Geometry: final body of the model. Coordinates: model frame, mm. A direction names the side the tool comes from. Round coordinates to 2 decimals unless told otherwise and drop trailing zeros. Write each loop counter-clockwise with the first axis right and the second up, starting at its lowest first coordinate (ties: lowest second). Pieces come first, ordered by that corner, then holes. Notation, with made-up numbers: M 61,20 L 106,20 A27 cw 106,38 Z; hole C 75.5,-35 d6. An arc over 180 degrees is marked long. Use one line per item in the form item = value. Start each with the question number.
Item 1: Pull-direction query (Z, two-part tool) for faces 1 (the flat face through (-27, 49, -12.5)), 2 (the flat face through (-1, 60, 10)), 3 (the flat face through (-1, 59.1, 0)), 4 (the flat face through (-27, 49, 12.5)); classes: pulls with the +Z half, pulls with the -Z half, needs draft (parallel to the pull), parting line crosses it, or undercut.
Item 2: Reachability of faces 5 (the flat face through (-60, -1, 0)), 6 (the cylindrical face through (58.797, 58.859, 9.712)), 7 (the flat face through (-56, 57, 0)), 8 (the flat face through (-0.3, 59.4, -7)), 9 (the flat face through (58, 55.1, 0)) from +Z, -Z, +X, -X, +Y, -Y: full face, straight path, thin tool, end or side. Return the list, or none.
Item 3: Ray query, probe 1 along Y at (x, z) = (15, -5.75); probe 2 along X at (y, z) = (50, -4.75); probe 3 along Y at (x, z) = (5, 11). Return the intervals inside material, ascending.
Item 4: Section query B-B (x = 0). Return loops of the section in (y, z), and give its area (3 significant figures).
Item 5: Pin query (flat end, axial travel): pin 1 Ø2 at (y, z) = (56.5, 2) entering from -X; pin 2 Ø4 at (x, y) = (-52.5, 52.5) entering from -Z; pin 3 Ø2 at (x, z) = (58.5, 0.5) entering from +Y; pin 4 Ø4 at (x, z) = (2.5, -4.5) entering from +Y. Return the tip coordinate at first contact, or that it passes through.
Item 6: Section query C-C (z = 5). Return loops of the section in (x, y), and give its area (3 significant figures).
Item 7: Section query D-D (x = 52.5). Return loops of the section in (y, z), and give its area (3 significant figures).
Item 8: Section query A-A (y = 0). Return loops of the section in (x, z), and give its area (3 significant figures).
Autodesk Inventor part; units mm, degrees
ref_plane "YZ Plane" through (0, 0, 0) normal (1, 0, 0) x (0, 1, 0)
ref_plane "XZ Plane" through (0, 0, 0) normal (0, 1, 0) x (-1, 0, 0)
ref_plane "XY Plane" through (0, 0, 0) normal (0, 0, 1) x (1, 0, 0)
sketch "Sketch1" plane through (0, 0, 0) normal (0, 0, 1) x (1, 0, 0)
  line L0 (-56, 60) -> (56, 60)
  line L1 (60, 56) -> (60, -56)
  line L2 (56, -60) -> (-56, -60)
  line L3 (-60, -56) -> (-60, 56)
  line L4 (-60, 60) -> (60, -60) construction
  line L5 (60, 60) -> (-60, -60) construction
  circle A0 centre (0, 0) radius 55
  line L6 (-52.5, 52.5) -> (52.5, 52.5) construction
  line L7 (52.5, 52.5) -> (52.5, -52.5) construction
  line L8 (52.5, -52.5) -> (-52.5, -52.5) construction
  line L9 (-52.5, -52.5) -> (-52.5, 52.5) construction
  line L10 (-52.5, 52.5) -> (52.5, -52.5) construction
  line L11 (52.5, 52.5) -> (-52.5, -52.5) construction
  circle A1 centre (-52.5, 52.5) radius 2.15
  circle A2 centre (-52.5, -52.5) radius 2.15
  circle A3 centre (52.5, -52.5) radius 2.15
  circle A4 centre (52.5, 52.5) radius 2.15
  arc A5 (-56, 60) -> (-60, 56) centre (-56, 56) ccw
  arc A6 (-60, -56) -> (-56, -60) centre (-56, -56) ccw
  arc A7 (56, -60) -> (60, -56) centre (56, -56) ccw
  arc A8 (60, 56) -> (56, 60) centre (56, 56) ccw
  dimension "d0" = 120
  dimension "d1" = 120
  dimension "d2" = 110
  dimension "d3" = 105
  dimension "d4" = 4.3
  dimension "d5" = 4.3
  dimension "d6" = 4.3
  dimension "d7" = 4.3
  dimension "d8" = 4
extrude "Extrusion1" add sketch "Sketch1" along normal mid plane 25
sketch "Sketch3" plane through (-56, 60, -12.5) normal (0, 1, 0) x (1, 0, 0)
  line L0 (-4, -5.5) -> (116, -5.5)
  line L1 (116, -5.5) -> (116, -19.5)
  line L2 (116, -19.5) -> (-4, -19.5)
  line L3 (-4, -19.5) -> (-4, -5.5)
  line L4 (-4, -5.5) -> (116, -19.5) construction
  line L5 (116, -5.5) -> (-4, -19.5) construction
  line L6 (-4, 0) -> (-4, -25)
  line L7 (116, 0) -> (116, -25)
  point P0 (56, -12.5)
  point P1 (-4, -12.5)
  dimension "d15" = 14
extrude "Extrusion3" cut sketch "Sketch3" against normal blind 0.9
sketch "Sketch4" plane through (-56, 59.1, -12.5) normal (0, 1, 0) x (1, 0, 0)
  line L0 (114.5278, -5.5) -> (114.5278, -19.5)
  line L1 (-2.5278, -5.5) -> (114.5278, -5.5)
  line L2 (-2.5278, -19.5) -> (-2.5278, -5.5)
  line L3 (114.5278, -19.5) -> (-2.5278, -19.5)
  line L4 (116, 0) -> (116, -25)
  line L5 (-4, 0) -> (-4, -25)
  line L6 (116, 0) -> (116, -25)
  line L7 (114.5278, -19.5) -> (-2.5278, -19.5)
  line L8 (116, -5.5) -> (112, -5.5)
  line L9 (112, -5.5) -> (112, -19.5)
  line L10 (112, -19.5) -> (116, -19.5)
  line L11 (116, -19.5) -> (116, -5.5)
  line L12 (-4, -5.5) -> (0, -5.5)
  line L13 (0, -5.5) -> (0, -19.5)
  line L14 (0, -19.5) -> (-4, -19.5)
  line L15 (-4, -19.5) -> (-4, -5.5)
  point P0 (56, -12.5)
  point P1 (116, -19.5)
  point P2 (116, -5.5)
  point P3 (-4, -19.5)
  point P4 (-2.5278, -19.5)
  dimension "d18" = 4
  dimension "d19" = 4
extrude "Extrusion4" cut sketch "Sketch4" against normal blind 4 contours L8 L4 L10 L0 | L0 L3 L9 L1 | L13 L3 L2 L1 | L2 L14 L5 L12
equation "\"d0\" = Size"
equation "\"d1\" = Size"
equation "\"d2\" = DuctDiammeter"
equation "\"d3\" = DistanceBetweenHoles"
equation "\"d8\" = CornerRadius"
equation "\"d9\" = Depth"
equation "\"Size\" = 120"
equation "\"DistanceBetweenHoles\" = 105"
equation "\"DuctDiammeter\" = 110"
equation "\"CornerRadius\" = 4"
equation "\"Depth\" = 25"
properties material "ABS Plastic"
Working result:
q1.face_1 = pulls with the -Z half
q1.face_2 = needs draft
q1.face_3 = undercut
q1.face_4 = pulls with the +Z half
q2.face_5 = +Z, -Z, -X, +Y, -Y
q2.face_6 = +Z, -Z, +X, +Y
q2.face_7 = -X, +Y
q2.face_8 = +Y
q2.face_9 = +X, +Y
q3.probe_1 = -60 to -52.92, 52.92 to 59.1
q3.probe_2 = -60 to -22.91, 22.91 to 60
q3.probe_3 = -60 to -54.77, 54.77 to 60
q4.outline = M -60,-12.5 L -55,-12.5 L -55,12.5 L -60,12.5 Z; M 55,-12.5 L 60,-12.5 L 60,-7 L 59.1,-7 L 59.1,7 L 60,7 L 60,12.5 L 55,12.5 Z
q4.area = 237 mm²
q5.pin_1 = -56
q5.pin_2 = through
q5.pin_3 = 55.1
q5.pin_4 = 59.1
q6.outline = M -60,-56 A4 ccw -56,-60 L 56,-60 A4 ccw 60,-56 L 60,55.1 L 56,55.1 L 56,59.1 L -56,59.1 L -56,55.1 L -60,55.1 Z; hole C 0,0 d110; hole C -52.5,-52.5 d4.3; hole C -52.5,52.5 d4.3; hole C 52.5,-52.5 d4.3; hole C 52.5,52.5 d4.3
q6.area = 4,690 mm²
q7.outline = M -60,-12.5 L -54.65,-12.5 L -54.65,12.5 L -60,12.5 Z; M -50.35,-12.5 L -16.39,-12.5 L -16.39,12.5 L -50.35,12.5 Z; M 16.39,-12.5 L 50.35,-12.5 L 50.35,12.5 L 16.39,12.5 Z; M 54.65,-12.5 L 60,-12.5 L 60,-7 L 59.1,-7 L 59.1,7 L 60,7 L 60,12.5 L 54.65,12.5 Z
q7.area = 1,950 mm²
q8.outline = M -60,-12.5 L -55,-12.5 L -55,12.5 L -60,12.5 Z; M 55,-12.5 L 60,-12.5 L 60,12.5 L 55,12.5 Z
q8.area = 250 mm²
